```python
from build123d import *

# Parameters (mm, degrees)
F0_R     = 3.302
F1_DEPTH = 6.35


with BuildPart() as f1:
    # F0 (on Top) → F1 (new body)
    with BuildSketch(Plane.XY):
        with BuildLine():
            ThreePointArc((-21.215855, 13.965941), (-7.289626, -24.331489), (25.4, 0))
            ThreePointArc((25.4, 0), (24.207914, 7.690052), (20.743551, 14.658278))
            ThreePointArc((20.743551, 14.658278), (-0.419047, 25.396543), (-21.215855, 13.965941))
        make_face()
        Circle(F0_R, mode=Mode.SUBTRACT)
        with BuildLine():
            ThreePointArc((-21.215855, 13.965941), (-0.419047, 25.396543), (20.743551, 14.658278))
            ThreePointArc((20.743551, 14.658278), (15.267392, 34.846937), (0, 49.146485))
            ThreePointArc((0, 49.146485), (-15.17191, 34.308552), (-21.215855, 13.965941))
        make_face()
    extrude(amount=F1_DEPTH)


solid = f1.part
```
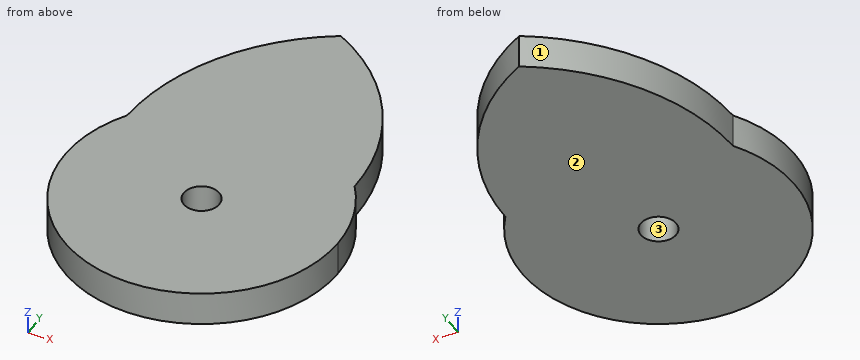
The listing builds one solid part. Answer for the finished solid, in the listing's coordinates (mm). Face numbers are marked on the shaded views. Give positions to 0.01 mm unless a question says otherwise; leave off trailing zeros. Write each loop counter-clockwise with the first axis right and the second up, starting at its lowest first coordinate (ties: lowest second). Pieces come first, ordered by that corner, then holes. Notation, with made-up numbers: (57.5, 24) - (96.5, 24) arc R19 cw to (96.5, 41) - close; hole circle Ø6 at (21, 72). An arc over 180 degrees is marked (long way). Use one line per item in the form item = value. Start each with the question number.
1) Flat-ended cylindrical pins translate along their axes: pin 1 Ø1 at (x, z) = (-2, 5.5) entering from +Y; pin 2 Ø2 at (y, z) = (2, 5) entering from +X; pin 3 Ø4 at (x, y) = (0, 0) entering from +Z. Find the tip coordinate at first contact, or state that the pin passes through.
2) Find section B-B on y = 2.5. Determine the outline of the cut face in (x, z), plus the area to 3 significant figures.
3) Consider line 1 along Y through (x, z) = (2, 0.75); line 2 along X through (y, z) = (25.5, 5.25); line 3 along X through (y, z) = (10, 4.75). Determine where each line is inside the solid, lowest interval first. Write a range as from..to.
4) Find section A-A on z = 2. Determine the outline of the cut face in (x, y).
5) Find section C-C on x = 17.5. Determine the outline of the cut face in (y, z), plus the area to 3 significant figures.
6) Find section D-D on y = 44.5. Determine the outline of the cut face in (x, z), plus the area to 3 significant figures.
7) The mould has two halves that part along X. Classify the marked faces 1, 2 and 3: pulls with the +X half, pulls with the -X half, needs draft (parallel to the pull), parting line crosses it, or undercut.
Geometry results:
q1.pin_1 = 48.25
q1.pin_2 = 25.38
q1.pin_3 = through
q2.outline = (-25.28, 0) - (-2.16, 0) - (-2.16, 6.35) - (-25.28, 6.35) - close; (2.16, 0) - (25.28, 0) - (25.28, 6.35) - (2.16, 6.35) - close
q2.area = 294 mm2
q3.line_1 = -25.32..-2.63, 2.63..48.04
q3.line_2 = -19.19..19.31
q3.line_3 = -23.35..23.35
q4.outline = (-21.22, 13.97) arc R25.4 ccw (long way) to (25.4, 0) arc R25.4 ccw to (20.74, 14.66) arc R38.3 ccw to (0, 49.15) arc R42.25 ccw to start; hole circle Ø6.6 at (0, 0)
q5.outline = (-18.41, 0) - (30.54, 0) - (30.54, 6.35) - (-18.41, 6.35) - close
q5.area = 311 mm2
q6.outline = (-6.57, 0) - (7, 0) - (7, 6.35) - (-6.57, 6.35) - close
q6.area = 86.2 mm2
q7.face_1 = pulls with the -X half
q7.face_2 = needs draft
q7.face_3 = undercut
